```python
from build123d import *

# Parameters (mm, degrees)
ESQUISSE1_W        = 6
ESQUISSE1_H        = 15
BOSS_EXTRU_1_DEPTH = 6


with BuildPart() as part:
    # Esquisse1 → Boss.-Extru.1 (new body)
    with BuildSketch(Plane.XY):
        Polygon((25.167583758, 47.381284916), (25.167583758, -12.618715084), (8.167583758, -12.618715084), (8.167583758, 47.381284916), (-7.832416242, 47.381284916), (-7.832416242, -12.618715084), (-24.832416242, -12.618715084), (-24.832416242, 47.381284916), (-40.832416242, 47.381284916), (-40.832416242, -72.618715084), (60.267583758, -72.618715084), (60.267583758, -22.618715084), (41.167583758, -22.618715084), (41.167583758, 47.381284916), align=None)
        with Locations((52.267583758, -62.118715084)):
            Rectangle(ESQUISSE1_W, ESQUISSE1_H, mode=Mode.SUBTRACT)
        with Locations((-11.732416242, -62.118715084)):
            Rectangle(ESQUISSE1_W, ESQUISSE1_H, mode=Mode.SUBTRACT)
    extrude(amount=BOSS_EXTRU_1_DEPTH)


solid = part.part
```
The model under review builds one solid part; all positions refer to its coordinate system, in mm. A direction names the side the tool comes from. Coordinates: 2 decimals unless noted, no trailing zeros. Write each loop counter-clockwise with the first axis right and the second up, starting at its lowest first coordinate (ties: lowest second). Pieces come first, ordered by that corner, then holes. Notation, with made-up numbers: (-34.5, 24) - (-22.5, 24) arc R27 cw to (-22.5, 45) - close; hole circle Ø7 at (13, 0.25). An arc over 180 degrees is marked (long way). Answer in a Markdown table with one row per item. Add a question column.
Q1. Consider section A-A on z = 1.9. Give the boundary of the cut face in (x, y).
Q2. Consider section D-D on y = 37.5. Give the boundary of the cut face in (x, z), then the cut area to 3 significant figures.
Q3. Consider section C-C on x = 51.5. Give the boundary of the cut face in (y, z), then the cut area to 3 significant figures.
Q4. Consider section B-B on y = -58. Give the boundary of the cut face in (x, z), then the cut area to 3 significant figures.
Q5. To check wall thickness, follow line 1 along X through (y, z) = (13, 4.85); line 2 along X through (y, z) = (-64, 2.1); line 3 along Y through (x, z) = (-12.5, 0.7). State the ranges of each line that lie inside material, in increasing order. Write a range as from..to.
Q6. For faces 4 (the face through (41.168, 12, 3)), 5 (the face through (60.268, -48, 3)), 6 (the face through (17, -12.619, 3)), 7 (the face through (49.268, -62, 3)), list the 3-axis set-ups (+Z, -Z, +X, -X, +Y, -Y) from which the entire face can be reached by the end or side of a thin tool; tool diameter is ignored.
Q7. Draft analysis for pull direction Y (two halves, no side actions). For faces 1 (the face through (0, 47.381, 3)), 2 (the face through (8.168, 17, 3)), 3 (the face through (52, -54.619, 3)), state which applies: +Y half, -Y half, draft (parallel to the pull), parting line (faces both ways), or undercut.
Q8. Clearance check with flat-ended pins moving along their axes: pin 1 (4 mm diameter, centred on x = 34, y = 16.5, fed in from -Z); pin 2 (3 mm diameter, centred on x = 51, z = 2, fed in from +Y); pin 3 (1.8 mm diameter, centred on x = 16, z = 3.5, fed in from +Y). State where each tip first meets the part, or that it passes through.
Answers below:
| question | item | result |
|---|---|---|
| 1 | outline | (-40.83, -72.62) - (60.27, -72.62) - (60.27, -22.62) - (41.17, -22.62) - (41.17, 47.38) - (25.17, 47.38) - (25.17, -12.62) - (8.17, -12.62) - (8.17, 47.38) - (-7.83, 47.38) - (-7.83, -12.62) - (-24.83, -12.62) - (-24.83, 47.38) - (-40.83, 47.38) - close; hole (-14.73, -69.62) - (-8.73, -69.62) - (-8.73, -54.62) - (-14.73, -54.62) - close; hole (49.27, -69.62) - (55.27, -69.62) - (55.27, -54.62) - (49.27, -54.62) - close |
| 2 | outline | (-40.83, 0) - (-24.83, 0) - (-24.83, 6) - (-40.83, 6) - close; (-7.83, 0) - (8.17, 0) - (8.17, 6) - (-7.83, 6) - close; (25.17, 0) - (41.17, 0) - (41.17, 6) - (25.17, 6) - close |
| 2 | area | 288 mm² |
| 3 | outline | (-72.62, 0) - (-69.62, 0) - (-69.62, 6) - (-72.62, 6) - close; (-54.62, 0) - (-22.62, 0) - (-22.62, 6) - (-54.62, 6) - close |
| 3 | area | 210 mm² |
| 4 | outline | (-40.83, 0) - (-14.73, 0) - (-14.73, 6) - (-40.83, 6) - close; (-8.73, 0) - (49.27, 0) - (49.27, 6) - (-8.73, 6) - close; (55.27, 0) - (60.27, 0) - (60.27, 6) - (55.27, 6) - close |
| 4 | area | 535 mm² |
| 5 | line 1 | -40.83..-24.83, -7.83..8.17, 25.17..41.17 |
| 5 | line 2 | -40.83..-14.73, -8.73..49.27, 55.27..60.27 |
| 5 | line 3 | -72.62..-69.62, -54.62..-12.62 |
| 6 | face 4 | +Z, -Z, +X, +Y |
| 6 | face 5 | +Z, -Z, +X, +Y, -Y |
| 6 | face 6 | +Z, -Z, +Y |
| 6 | face 7 | +Z, -Z |
| 7 | face 1 | +Y half |
| 7 | face 2 | draft |
| 7 | face 3 | undercut |
| 8 | pin 1 | z = 0 |
| 8 | pin 2 | y = -22.62 |
| 8 | pin 3 | y = -12.62 |
